Model file for the job. Use its own axes, mm. A direction names the side the tool comes from. Give positions to 0.01 mm unless a question says otherwise; leave off trailing zeros. Loops run counter-clockwise (first coordinate to the right, second up) from the corner with the lowest first, then second, coordinate; pieces in that order, holes last. Notation, with made-up numbers: M 30,84 L 78,84 A31 ccw 78,112 Z; hole C -36,58.5 d9. An arc over 180 degrees is marked long. Answer in a Markdown table with one row per item.
```python
from build123d import *

# Parameters (mm, degrees)
BOSS_EXTRUDE1_DEPTH = 3
SKETCH2_R           = 1
BOSS_EXTRUDE2_DEPTH = 3
SKETCH3_R           = 1
BOSS_EXTRUDE3_DEPTH = 3


with BuildPart() as part:
    # Sketch1 → Boss-Extrude1 (new body)
    with BuildSketch(Plane.XY):
        with BuildLine():
            Line((-10.074027202, 4.819774295), (-8.80607801, 4.819774295))
            ThreePointArc((-8.80607801, 4.819774295), (-5.074027202, 3.819774295), (-8.80607801, 2.819774295))
            Line((-8.80607801, 2.819774295), (-10.074027202, 2.819774295))
            ThreePointArc((-10.074027202, 2.819774295), (-11.074027202, 3.819774295), (-10.074027202, 4.819774295))
        make_face()
    extrude(amount=BOSS_EXTRUDE1_DEPTH)

    # Sketch2 → Boss-Extrude2 (add)
    with BuildSketch(Plane.XY.offset(3)):
        with Locations((-10.074027202, 3.819774295)):
            Circle(SKETCH2_R)
    extrude(amount=BOSS_EXTRUDE2_DEPTH)

    # Sketch3 → Boss-Extrude3 (add)
    with BuildSketch(Plane(origin=(0, 0, 0), x_dir=(-1, 0, 0), z_dir=(0, 0, -1))):
        with Locations((7.074027202, 3.819774295)):
            Circle(SKETCH3_R)
    extrude(amount=BOSS_EXTRUDE3_DEPTH)


solid = part.part
```
(1) Which spindle directions (+Z, -Z, +X, -X, +Y, -Y) get a long thin tool onto all of the face, cutting with end or side? Do faces 1 (the flat face through (-9, 2.82, 1)), 2 (the flat face through (-9, 4.82, 1)), 3 (the cylindrical face through (-8.028, 4.12, -1.479)), 4 (the cylindrical face through (-5.075, 3.893, 1.479)). Say none if no direction does.
Established:
| item | result |
|---|---|
| face 1 | +Z, -Z, -X, -Y |
| face 2 | +Z, -Z, -X, +Y |
| face 3 | -Z |
| face 4 | +Z, -Z |
(2) Saw through at A-A, the plane y = 3.3. Give the cut face in (x, z), and give its area (3 significant figures).
Established:
| item | result |
|---|---|
| outline | M -10.93,0 L -7.93,0 L -7.93,-3 L -6.22,-3 L -6.22,0 L -5.14,0 L -5.14,3 L -9.22,3 L -9.22,6 L -10.93,6 Z |
| area | 27.6 mm2 |
(3) Flat gauge pins, fed straight in: P1, Ø1.2, axis at x = -8, y = 3, coming from the +Z side; P2, Ø3, axis at x = -10, z = 4.5, coming from the +Y side; P3, Ø1.5, axis at y = 2.5, z = -0.5, coming from the +X side. Where does each tip first touch, or does it go through?
Established:
| item | result |
|---|---|
| P1 | stops at z = 3 |
| P2 | stops at y = 4.82 |
| P3 | stops at x = -5.22 |
(4) Wall check: L1, parallel to Y at x = -10.1, z = 4.75; L2, parallel to Z at x = -8.2, y = 5.1; L3, parallel to Y at x = -10.5, z = 0.75. Give the ranges that are in metal, low to high.
Established:
| item | result |
|---|---|
| L1 | y = 2.82 to 4.82 |
| L2 | z = 0 to 3 |
| L3 | y = 2.92 to 4.72 |
(5) Saw through at C-C, the plane z = 1. Give the cut face in (x, y), and give its area (3 significant figures).
Established:
| item | result |
|---|---|
| outline | M -10.07,2.82 L -8.81,2.82 A2 ccw long -8.81,4.82 L -10.07,4.82 A1 ccw Z |
| area | 16.3 mm2 |
(6) Saw through at D-D, the plane x = -6.65. Give the cut face in (y, z).
Established:
| item | result |
|---|---|
| outline | M 1.87,0 L 2.91,0 L 2.91,-3 L 4.73,-3 L 4.73,0 L 5.77,0 L 5.77,3 L 1.87,3 Z |
